```python
from build123d import *


with BuildPart() as part:
    # Эскиз1 → Повернуть1 (revolve)
    with BuildSketch(Plane.XY):
        with BuildLine():
            Line((1.5, 31), (0.27515818, 33.819532322))
            ThreePointArc((0.27515818, 33.819532322), (0.164530094, 33.950858224), (0, 34))
            Line((0, 34), (0, 32))
            ThreePointArc((0, 32), (0.353553391, 31.853553391), (0.5, 31.5))
            Line((0.5, 31.5), (0.5, 10.153882032))
            ThreePointArc((0.5, 10.153882032), (0.614241625, 9.835777527), (0.904761905, 9.663036124))
            ThreePointArc((0.904761905, 9.663036124), (4.728209047, 4.545534154), (0, 0.25))
            Line((0, 0.25), (0, 0))
            ThreePointArc((0, 0), (4.913681129, 4.074939047), (1.818181818, 9.657704894))
            ThreePointArc((1.818181818, 9.657704894), (1.587138588, 9.841437346), (1.5, 10.123475383))
            Line((1.5, 10.123475383), (1.5, 31))
        make_face()
    revolve(axis=Axis((0, 0, 0), (0, 1, 0)))


solid = part.part
```
Could you check a few things on this model? Use its own coordinates, in mm. Give positions to 0.01 mm unless a question says otherwise; leave off trailing zeros. Order: outer loops, then holes, each group sorted by start corner. A loop starts at its lowest first (then second) coordinate and runs counter-clockwise, first axis right, second up.
Q1. If I drill on line 1 along Z through (x, y) = (0, 26.5); line 2 along Y through (x, z) = (0, 4), over which ranges is the centre line in solid material (lowest first)?
Q2. We'd pull the mould along X, two halves only. Please class faces 1 (the cylindrical face through (-0.108, 20.678, 0.488)), 2 (the conical face through (-0.59, 32.74, 0.45)): +X half, -X half, draft (parallel to the pull), parting line (faces both ways), or undercut.
Q3. Suppose I cut it at B-B, the plane x = -3.75. Write out the boundary of the cut face in (y, z).
Q4. Suppose I cut it at A-A, the plane y = 5. Write out the boundary of the cut face in (x, z).
Q5. I'm going to push flat-ended pins straight in: P1, Ø1.5, axis at y = 30.5, z = -1, coming from the +X side; P2, Ø1, axis at x = -3.5, z = 0.5, coming from the +Y side; P3, Ø5, axis at x = 1.5, y = 24, coming from the +Z side. Where does each tip first touch, or does it pass through?
Solution:
1. line 1: z = -1.5 to -0.5, 0.5 to 1.5
1. line 2: y = 2 to 2.44, 7.56 to 8
2. face 1: undercut
2. face 2: parting line
3. outline: circle Ø6.61 at (5, 0); hole circle Ø5.83 at (5, 0)
4. outline: circle Ø10 at (0, 0); hole circle Ø9.5 at (0, 0)
5. P1: stops at x = 1.48
5. P2: stops at y = 8.97
5. P3: stops at z = 1.5
